Check sheet for the drawn part. Datum: minimum x, y, z corner. Units: mm. Round coordinates to 2 decimals unless told otherwise and drop trailing zeros. Order: outer loops, then holes, each group sorted by start corner. A loop starts at its lowest first (then second) coordinate and runs counter-clockwise, first axis right, second up. Notation, with made-up numbers: (-36, 61) - (-2, 61) arc R5 ccw to (-2, 69) - close; hole circle Ø10 at (52, 22). An arc over 180 degrees is marked (long way). Write each question's results on one line, items separated by ' | '.
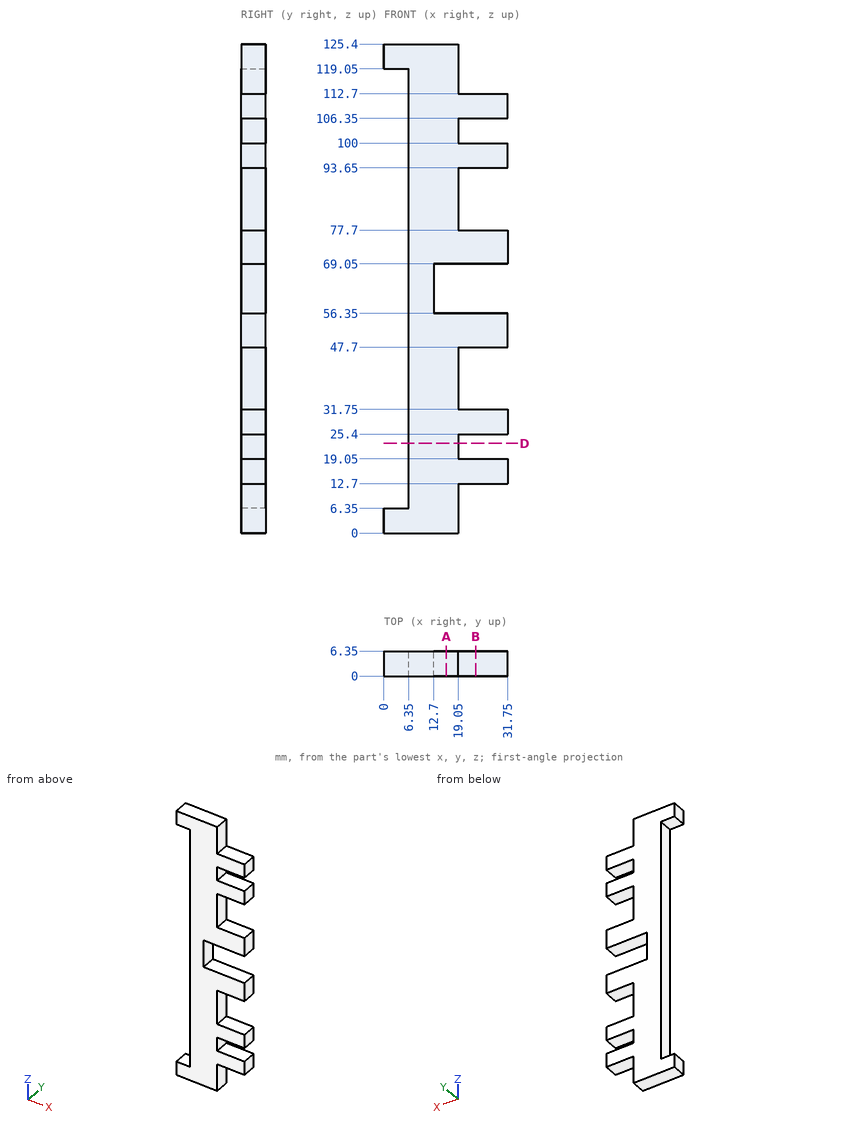
(1) Material ranges on line 1 (Z direction, x = 20, y = 1); line 2 (Z direction, x = 16, y = 2.5); line 3 (X direction, y = 2.5, z = 92.5), recorded low to high.
Answers follow:
line 1: 12.7 to 19.05, 25.4 to 31.75, 47.7 to 56.35, 69.05 to 77.7, 93.65 to 100, 106.35 to 112.7 | line 2: 0 to 56.35, 69.05 to 125.4 | line 3: 6.35 to 19.05
(2) Section check D-D (z = 23). Record the cut outline in (x, y), then the cut area to 3 significant figures.
Answers follow:
outline: (6.35, 0) - (19.05, 0) - (19.05, 6.35) - (6.35, 6.35) - close | area: 80.6 mm²
(3) Section check B-B (x = 23.5). Record the cut outline in (y, z).
Answers follow:
outline: (0, 12.7) - (6.35, 12.7) - (6.35, 19.05) - (0, 19.05) - close; (0, 25.4) - (6.35, 25.4) - (6.35, 31.75) - (0, 31.75) - close; (0, 47.7) - (6.35, 47.7) - (6.35, 56.35) - (0, 56.35) - close; (0, 69.05) - (6.35, 69.05) - (6.35, 77.7) - (0, 77.7) - close; (0, 93.65) - (6.35, 93.65) - (6.35, 100) - (0, 100) - close; (0, 106.35) - (6.35, 106.35) - (6.35, 112.7) - (0, 112.7) - close
(4) Depth check by flat-ended pin: pin 1 Ø3 at (y, z) = (2.5, 21.5) entering from +X; pin 2 Ø3 at (x, y) = (28, 2) entering from +Z; pin 3 Ø1.9 at (x, y) = (23.5, 2.5) entering from -Z. Enter the tip coordinate at first touch or a pass-through.
Answers follow:
pin 1: x = 19.05 | pin 2: z = 112.7 | pin 3: z = 12.7
(5) Section check A-A (x = 16). Record the cut outline in (y, z), then the cut area to 3 significant figures.
Answers follow:
outline: (0, 0) - (6.35, 0) - (6.35, 56.35) - (0, 56.35) - close; (0, 69.05) - (6.35, 69.05) - (6.35, 125.4) - (0, 125.4) - close | area: 716 mm²
